Check sheet for the modelled part. Datum: model origin and axes. Units: mm. A direction names the side the tool comes from. Round coordinates to 2 decimals unless told otherwise and drop trailing zeros. Order: outer loops, then holes, each group sorted by start corner. A loop starts at its lowest first (then second) coordinate and runs counter-clockwise, first axis right, second up.
Q1. Scan lines: probe 1 along X at (y, z) = (87, 0); probe 2 along X at (y, z) = (96, -4); probe 3 along Y at (x, z) = (-16, -46.5). Record each from-to range of solid material in increasing order.
Q2. Set-up check for faces 4 (the flat face through (73, 0, -4)), 5 (the flat face through (1, 136, 1)): record each of +Z, -Z, +X, -X, +Y, -Y from which the full face is reachable in a straight line by a thin tool's end or side.
Q3. Cross-section at D-D on y = 247. Record the cut outline in (x, z).
Q4. Cross-section at A-A on x = 0. Record the cut outline in (y, z).
Q5. Depth check by flat-ended pin: P1, Ø5, axis at x = 212, y = 170.5, coming from the -Z side; P2, Ø2, axis at x = 186, y = 136.5, coming from the +Z side; P3, Ø10, axis at x = 241.5, y = 93, coming from the -Z side; P4, Ø4, axis at x = -4.5, z = -236.5, coming from the -Y side. Enter the tip coordinate at first touch or a pass-through.
Q6. Cross-section at B-B on z = 0. Record the cut outline in (x, y).
Q7. Mould release check, pull along X, two halves, no side actions. Record for faces 1 (the cylindrical face through (-340.945, 175.871, -75.711)), 2 (the flat face through (4, 355.6, -4)), 3 (the cylindrical face through (19.674, 67.048, -62.475)): +X half, -X half, draft (parallel to the pull), parting line (faces both ways), or undercut.
Q8. Cross-section at C-C on y = 117. Record the cut outline in (x, z), then the cut area to 3 significant figures.
from build123d import *

# Parameters (mm, degrees)
SCHIZZO1_R                   = 349.25
ESTRUSIONE_ESTRUSIONE1_DEPTH = 355.6
RACCORDO1_R                  = 40
SCHIZZO2_R                   = 65.5
TAGLIO_ESTRUSIONE1_DEPTH     = 136


with BuildPart() as part:
    # Schizzo1 → Estrusione-Estrusione1 (new body)
    with BuildSketch(Plane(origin=(0, 0, 0), x_dir=(-1, 0, 0), z_dir=(0, 1, 0))):
        with Locations(Location((0, 0, 0), (0, 0, 90))):
            Circle(SCHIZZO1_R)
    extrude(amount=ESTRUSIONE_ESTRUSIONE1_DEPTH)

    # Raccordo1
    raccordo1_edges = [part.edges().sort_by_distance(p)[0] for p in [
        (0, 0, -349.25),
        (0, 355.6, -349.25),
    ]]
    fillet(raccordo1_edges, radius=RACCORDO1_R)

    # Schizzo2 → Taglio-Estrusione1 (cut)
    with BuildSketch(Plane.XZ):
        with Locations(Location((0, 0, 0), (0, 0, 270))):
            Circle(SCHIZZO2_R)
    extrude(amount=-TAGLIO_ESTRUSIONE1_DEPTH, mode=Mode.SUBTRACT)


solid = part.part
Results found:
1. probe 1: x = -349.25 to -65.5, 65.5 to 349.25
1. probe 2: x = -349.23 to -65.38, 65.38 to 349.23
1. probe 3: y = 136 to 355.6
2. face 4: +Z, -Z, +X, -X, -Y
2. face 5: -Y
3. outline: circle Ø698.5 at (0, 0)
4. outline: (0, -309.25) arc R40 ccw to (40, -349.25) - (315.6, -349.25) arc R40 ccw to (355.6, -309.25) - (355.6, 309.25) arc R40 ccw to (315.6, 349.25) - (40, 349.25) arc R40 ccw to (0, 309.25) - (0, 65.5) - (136, 65.5) - (136, -65.5) - (0, -65.5) - close
5. P1: stops at z = -279.44
5. P2: stops at z = 296.23
5. P3: stops at z = -256.99
5. P4: stops at y = 0
6. outline: (-349.25, 40) arc R40 ccw to (-309.25, 0) - (-65.5, 0) - (-65.5, 136) - (65.5, 136) - (65.5, 0) - (309.25, 0) arc R40 ccw to (349.25, 40) - (349.25, 315.6) arc R40 ccw to (309.25, 355.6) - (-309.25, 355.6) arc R40 ccw to (-349.25, 315.6) - close
7. face 1: parting line
7. face 2: draft
7. face 3: undercut
8. outline: circle Ø698.5 at (0, 0); hole circle Ø131 at (0, 0)
8. area: 370,000 mm2
